Design review of the part built by this model. Coordinates are the model's own, in mm. Round coordinates to 2 decimals unless told otherwise and drop trailing zeros. Order: outer loops, then holes, each group sorted by start corner. A loop starts at its lowest first (then second) coordinate and runs counter-clockwise, first axis right, second up. Notation, with made-up numbers: (20, 15) - (68, 15) arc R27 ccw to (68, 52) - close; hole circle Ø10 at (29, 22). An arc over 180 degrees is marked (long way). Use CSV: the item, a comma, the result in double quotes.
from build123d import *

# Parameters (mm, degrees)
SKETCH1_R           = 35
BOSS_EXTRUDE1_DEPTH = 15
SKETCH2_R           = 20
CUT_EXTRUDE1_DEPTH  = 3
FILLET2_R           = 2
SKETCH4_R           = 2.5
CUT_EXTRUDE2_DEPTH  = 51.931326313
CUT_EXTRUDE3_DEPTH  = 51.931326313
FILLET3_R           = 5


with BuildPart() as part:
    # Sketch1 → Boss-Extrude1 (new body)
    with BuildSketch(Plane.XY):
        Circle(SKETCH1_R)
    extrude(amount=BOSS_EXTRUDE1_DEPTH)

    # Sketch2 → Cut-Extrude1 (cut)
    with BuildSketch(Plane(origin=(0, 0, 0), x_dir=(-1, 0, 0), z_dir=(0, 0, -1))):
        Circle(SKETCH2_R)
    extrude(amount=-CUT_EXTRUDE1_DEPTH, mode=Mode.SUBTRACT)

    # Fillet2
    fillet2_edges = [part.edges().sort_by_distance(p)[0] for p in [
        (20, 0, 3),
    ]]
    fillet(fillet2_edges, radius=FILLET2_R)

    # Sketch4 → Cut-Extrude2 (cut, through all)
    with BuildSketch(Plane(origin=(0, 0, 3), x_dir=(-1, 0, 0), z_dir=(0, 0, -1))):
        Circle(SKETCH4_R)
    extrude(amount=-CUT_EXTRUDE2_DEPTH, mode=Mode.SUBTRACT)

    # Sketch5 → Cut-Extrude3 (cut, through all)
    with BuildSketch(Plane(origin=(0, 0, 3), x_dir=(-1, 0, 0), z_dir=(0, 0, -1))):
        with BuildLine():
            Line((0, 5), (0, 18))
            ThreePointArc((0, 18), (4.658742812, 17.386664873), (9, 15.588457268))
            Line((9, 15.588457268), (2.5, 4.330127019))
            ThreePointArc((2.5, 4.330127019), (1.294095226, 4.829629131), (0, 5))
        make_face()
        with BuildLine():
            Line((4.890738004, -1.039558454), (17.606656813, -3.742410435))
            ThreePointArc((17.606656813, -3.742410435), (17.975331626, 0.942047212), (17.119017293, 5.562305899))
            Line((17.119017293, 5.562305899), (4.755282581, 1.545084972))
            ThreePointArc((4.755282581, 1.545084972), (4.993147674, 0.261679781), (4.890738004, -1.039558454))
        make_face()
        with BuildLine():
            Line((0.522642316, -4.972609477), (1.881512339, -17.901394117))
            ThreePointArc((1.881512339, -17.901394117), (6.450623092, -16.804447677), (10.580134541, -14.562305899))
            Line((10.580134541, -14.562305899), (2.938926261, -4.045084972))
            ThreePointArc((2.938926261, -4.045084972), (1.791839748, -4.667902132), (0.522642316, -4.972609477))
        make_face()
        with BuildLine():
            Line((-4.567727288, -2.033683215), (-16.443818238, -7.321259575))
            ThreePointArc((-16.443818238, -7.321259575), (-13.988627306, -11.327767039), (-10.580134541, -14.562305899))
            Line((-10.580134541, -14.562305899), (-2.938926261, -4.045084972))
            ThreePointArc((-2.938926261, -4.045084972), (-3.885729807, -3.146601955), (-4.567727288, -2.033683215))
        make_face()
        with BuildLine():
            Line((-3.345653032, 3.715724127), (-12.044350914, 13.376606859))
            ThreePointArc((-12.044350914, 13.376606859), (-15.096070223, 9.80350263), (-17.119017293, 5.562305899))
            Line((-17.119017293, 5.562305899), (-4.755282581, 1.545084972))
            ThreePointArc((-4.755282581, 1.545084972), (-4.19335284, 2.723195175), (-3.345653032, 3.715724127))
        make_face()
    extrude(amount=-CUT_EXTRUDE3_DEPTH, mode=Mode.SUBTRACT)

    # Fillet3
    fillet3_edges = [part.edges().sort_by_distance(p)[0] for p in [
        (-35, 0, 0),
    ]]
    fillet(fillet3_edges, radius=FILLET3_R)


solid = part.part
1) Insertion check: pin 1 Ø5 at (x, z) = (-1, 7) entering from -Y; pin 2 Ø6.5 at (x, y) = (0, 0) entering from -Z; pin 3 Ø3 at (y, z) = (-3.5, 13.5) entering from -X. Each pin has a flat end and moves straight along its axis. Give the tip position at first contact, or say it passes through.
Data:
pin 1,"stops at y = -35"
pin 2,"stops at z = 3"
pin 3,"stops at x = -34.94"
2) To check wall thickness, follow L1, parallel to X at y = -10, z = 10.5; L2, parallel to X at y = -13.5, z = 8; L3, parallel to Z at x = 3, y = 0.5. State the ranges of each line that lie inside material, in increasing order. Write a range as from..to.
Data:
L1,"x = -33.54..-7.27, -1.05..7.27, 14.97..33.54"
L2,"x = -32.29..-9.81, -1.42..9.81, 11.91..32.29"
L3,"z = 3..15"
3) The part is to be moulded in two halves that separate along Y. For faces 1 (the face through (10.42, -4.64, 8.92)), 2 (the face through (-1.81, -4.66, 8.92)), 3 (the face through (-28, -21, 10)), say which applies: +Y half, -Y half, draft (parallel to the pull), parting line (faces both ways), or undercut.
Data:
face 1,"undercut"
face 2,"undercut"
face 3,"parting line"
4) We need section B-B (z = 13). Give the boundary of the cut face in (x, y), then the cut area to 3 significant figures.
Data:
outline,"circle Ø70 at (0, 0); hole (-17.61, -3.74) - (-4.89, -1.04) arc R5 cw to (-4.76, 1.55) - (-17.12, 5.56) arc R18 ccw to start; hole (-10.58, -14.56) arc R18 ccw to (-1.88, -17.9) - (-0.52, -4.97) arc R5 cw to (-2.94, -4.05) - close; hole (-9, 15.59) - (-2.5, 4.33) arc R5 cw to (0, 5) - (0, 18) arc R18 ccw to start; hole circle Ø5 at (0, 0); hole (2.94, -4.05) - (10.58, -14.56) arc R18 ccw to (16.44, -7.32) - (4.57, -2.03) arc R5 cw to start; hole (3.35, 3.72) arc R5 cw to (4.76, 1.55) - (17.12, 5.56) arc R18 ccw to (12.04, 13.38) - close"
area,"3,440 mm2"
5) We need section A-A (y = 0). Give the boundary of the cut face in (x, z), then the cut area to 3 significant figures.
Data:
outline,"(-35, 5) arc R5 ccw to (-30, 0) - (-20, 0) - (-20, 1) arc R2 cw to (-18, 3) - (-18, 15) - (-35, 15) - close; (-5, 3) - (-2.5, 3) - (-2.5, 15) - (-5, 15) - close; (2.5, 3) - (18, 3) arc R2 cw to (20, 1) - (20, 0) - (30, 0) arc R5 ccw to (35, 5) - (35, 15) - (2.5, 15) - close"
area,"705 mm2"
6) We need section C-C (x = 9). Give the number of separate pieces and of enclosed holes in the cut face, then the cut area to 3 significant figures.
Data:
separate pieces,"3"
enclosed holes,"0"
area,"713 mm2"
